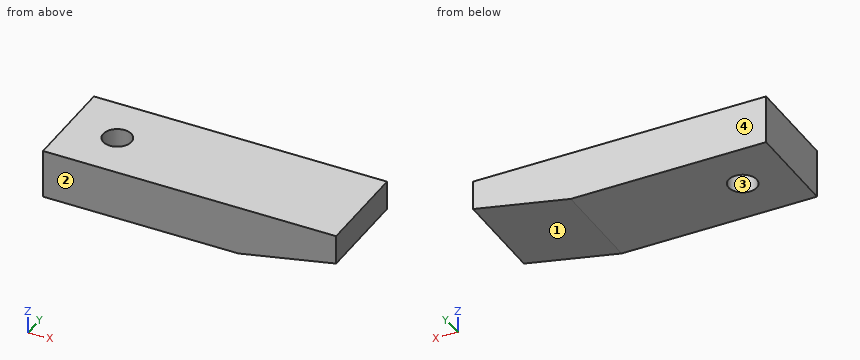
```python
from build123d import *

# Parameters (mm, degrees)
SKETCH1_W                   = 38.1
SKETCH1_H                   = 6.35
BOSS_EXTRUDE1_DEPTH         = 6.35
F_27_0_144_DIAMETER_HOLE1_D = 3.6576
CUT_EXTRUDE1_DEPTH          = 13.7


with BuildPart() as part:
    # Sketch1 → Boss-Extrude1 (new body, symmetric)
    with BuildSketch(Plane(origin=(0, 0, 0), x_dir=(-1, 0, 0), z_dir=(0, 1, 0))):
        Rectangle(SKETCH1_W, SKETCH1_H)
    extrude(amount=BOSS_EXTRUDE1_DEPTH, both=True)

    # #27 (0.144) Diameter Hole1 (through all)
    with Locations(Plane.XY.offset(3.175)):
        with Locations((-12.7, 0)):
            Hole(F_27_0_144_DIAMETER_HOLE1_D / 2)

    # Sketch5 → Cut-Extrude1 (cut, through all)
    with BuildSketch(Plane.XZ.offset(6.35)):
        Polygon((19.05, -0.635), (6.35, -3.175), (19.05, -3.175), align=None)
    extrude(amount=-CUT_EXTRUDE1_DEPTH, mode=Mode.SUBTRACT)


solid = part.part
```
Design review of the part built by this model. Coordinates are the model's own, in mm. Face numbers are marked on the shaded views. Give positions to 0.01 mm unless a question says otherwise; leave off trailing zeros. Order: outer loops, then holes, each group sorted by start corner. A loop starts at its lowest first (then second) coordinate and runs counter-clockwise, first axis right, second up. Notation, with made-up numbers: M 3,10.25 L 38,10.25 A31 cw 38,36.25 Z; hole C -21,50 d11. An arc over 180 degrees is marked long. One line per question, with ' | ' between items. Start each with the question number.
Q1. The part is to be moulded in two halves that separate along Y. For the marked faces 1, 2, 3 and 4, say which applies: +Y half, -Y half, draft (parallel to the pull), parting line (faces both ways), or undercut.
Q2. For pin 1 Ø3 at (x, y) = (-12.7, 0) entering from +Z, flat-tipped, find the tip position at first contact; note if it passes through.
Q3. We need section B-B (x = -12.7). Write out the cut boundary in (y, z) (3 decimals), plus the area to 3 significant figures.
Q4. For L1, parallel to Y at x = -12.7, z = 1; L2, parallel to X at y = -0.75, z = 2.75; L3, parallel to X at y = -0.5, z = 2.5, list the stretches that pass through material, from the lowest coordinate up. Write a range as [from, to].
Q5. We need section A-A (y = 0). Write out the cut boundary in (x, z) (3 decimals), plus the area to 3 significant figures.
Q6. We need section D-D (y = -3.25). Write out the cut boundary in (x, z) (3 decimals), plus the area to 3 significant figures.
Q7. We need section C-C (z = 0). Write out the cut boundary in (x, y).
Returned:
1) face 1: draft | face 2: -Y half | face 3: undercut | face 4: +Y half
2) pin 1: through
3) outline: M -6.35,-3.175 L -1.829,-3.175 L -1.829,3.175 L -6.35,3.175 Z; M 1.829,-3.175 L 6.35,-3.175 L 6.35,3.175 L 1.829,3.175 Z | area: 57.4 mm2
4) L1: [-6.35, -1.83], [1.83, 6.35] | L2: [-19.05, -14.37], [-11.03, 19.05] | L3: [-19.05, -14.46], [-10.94, 19.05]
5) outline: M -19.05,-3.175 L -14.529,-3.175 L -14.529,3.175 L -19.05,3.175 Z; M -10.871,-3.175 L 6.35,-3.175 L 19.05,-0.635 L 19.05,3.175 L -10.871,3.175 Z | area: 203 mm2
6) outline: M -19.05,-3.175 L 6.35,-3.175 L 19.05,-0.635 L 19.05,3.175 L -19.05,3.175 Z | area: 226 mm2
7) outline: M -19.05,-6.35 L 19.05,-6.35 L 19.05,6.35 L -19.05,6.35 Z; hole C -12.7,0 d3.66
